For this review, take the finished solid that the model builds, in its own axes (mm). A direction names the side the tool comes from. Coordinates: 2 decimals unless noted, no trailing zeros. Loops run counter-clockwise (first coordinate to the right, second up) from the corner with the lowest first, then second, coordinate; pieces in that order, holes last. Notation, with made-up numbers: M 6.25,-8 L 13.25,-8 A32 cw 13.25,18 Z; hole C 79.5,63 d6. An arc over 180 degrees is marked long. Write each question's results on one line, items separated by ' | '. Start each with the question number.
```python
from build123d import *

# Parameters (mm, degrees)
EXTRUDE_1_DEPTH     = 39.9
SKETCH_2_R          = 1.5
CUT_EXTRUDE_1_DEPTH = 3
CHAMFER_1_SIZE      = 0.5


with BuildPart() as part:
    # 草图1 → 凸台-拉伸1 (new body)
    with BuildSketch(Plane(origin=(0, 0, 0), x_dir=(1, 0, 0), z_dir=(0, 1, 0))):
        Polygon((-10, 4), (-10, -4), (-4.5, -4), (-4.5, -2.84), (-3.55, -2.84), (-3.55, -1.36), (-4.5, -1.36), (-4.5, 0), (4.5, 0), (4.5, -1.36), (3.55, -1.36), (3.55, -2.84), (4.5, -2.84), (4.5, -4), (10, -4), (10, 4), align=None)
    extrude(amount=EXTRUDE_1_DEPTH)

    # 草图2 → 切除-拉伸1 (cut)
    with BuildSketch(Plane(origin=(0, 0, -4), x_dir=(-1, 0, 0), z_dir=(0, 0, -1))):
        with Locations((7.5, 27.95)):
            Circle(SKETCH_2_R)
        with Locations(Location((-7.5, 27.95, 0), (0, 0, 180))):
            Circle(SKETCH_2_R)
        with Locations(Location((7.5, 11.95, 0), (0, 0, 180))):
            Circle(SKETCH_2_R)
        with Locations((-7.5, 11.95)):
            Circle(SKETCH_2_R)
    extrude(amount=-CUT_EXTRUDE_1_DEPTH, mode=Mode.SUBTRACT)

    # 倒角1
    chamfer_1_edges = [part.edges().sort_by_distance(p)[0] for p in [
        (-10, 19.95, 4),
        (-10, 19.95, -4),
        (10, 19.95, -4),
        (10, 19.95, 4),
    ]]
    chamfer(chamfer_1_edges, length=CHAMFER_1_SIZE)


solid = part.part
```
Q1. To check wall thickness, follow line 1 along Y through (x, z) = (-7.5, -2.3); line 2 along X through (y, z) = (35, 1); line 3 along Z through (x, y) = (-3, 20). State the ranges of each line that lie inside material, in increasing order.
Q2. Take a section at C-C, the plane x = 7.5. Give the boundary of the cut face in (y, z), then the cut area to 3 significant figures.
Q3. For faces 4 (the face through (-3.55, 20, 2)), 5 (the face through (-8.69, 12.86, -2.52)), 6 (the face through (-4.5, 20, 1)), list the 3-axis set-ups (+Z, -Z, +X, -X, +Y, -Y) from which the entire face can be reached by the end or side of a thin tool; tool diameter is ignored.
Q4. Take a section at A-A, the plane z = -2.25. Give the boundary of the cut face in (x, y), then the cut area to 3 significant figures.
Q5. Insertion check: P1, Ø10, axis at x = -0.5, y = 21, coming from the +Z side; P2, Ø2.5, axis at x = -7.5, y = 11.95, coming from the -Z side. Each pin has a flat end and moves straight along its axis. Give the tip position at first contact, or say it passes through.
Q6. The part is to be moulded in two halves that separate along X. For faces 1 (the face through (7, 20, 4)), 2 (the face through (10, 20, 0)), 3 (the face through (-4.5, 20, 3)), say which applies: pulls with the +X half, pulls with the -X half, needs draft (parallel to the pull), parting line crosses it, or undercut.
Q7. Take a section at D-D, the plane y = 11. Give the boundary of the cut face in (x, z).
Q8. Take a section at B-B, the plane y = 24. Give the boundary of the cut face in (x, z).
Results:
1) line 1: 0 to 10.45, 13.45 to 26.45, 29.45 to 39.9 | line 2: -10 to -4.5, 4.5 to 10 | line 3: -4 to 0
2) outline: M 0,-4 L 10.45,-4 L 10.45,-1 L 13.45,-1 L 13.45,-4 L 26.45,-4 L 26.45,-1 L 29.45,-1 L 29.45,-4 L 39.9,-4 L 39.9,4 L 0,4 Z | area: 301 mm^2
3) face 4: +Z, +Y, -Y | face 5: -Z | face 6: +Y, -Y
4) outline: M -10,0 L 10,0 L 10,39.9 L -10,39.9 Z; hole C -7.5,11.95 d3; hole C -7.5,27.95 d3; hole C 7.5,11.95 d3; hole C 7.5,27.95 d3 | area: 770 mm^2
5) P1: z = 4 | P2: z = -1
6) face 1: needs draft | face 2: pulls with the +X half | face 3: undercut
7) outline: M -10,-3.5 L -9.5,-4 L -8.66,-4 L -8.66,-1 L -6.34,-1 L -6.34,-4 L 6.34,-4 L 6.34,-1 L 8.66,-1 L 8.66,-4 L 9.5,-4 L 10,-3.5 L 10,3.5 L 9.5,4 L 4.5,4 L 4.5,2.84 L 3.55,2.84 L 3.55,1.36 L 4.5,1.36 L 4.5,0 L -4.5,0 L -4.5,1.36 L -3.55,1.36 L -3.55,2.84 L -4.5,2.84 L -4.5,4 L -9.5,4 L -10,3.5 Z
8) outline: M -10,-3.5 L -9.5,-4 L 9.5,-4 L 10,-3.5 L 10,3.5 L 9.5,4 L 4.5,4 L 4.5,2.84 L 3.55,2.84 L 3.55,1.36 L 4.5,1.36 L 4.5,0 L -4.5,0 L -4.5,1.36 L -3.55,1.36 L -3.55,2.84 L -4.5,2.84 L -4.5,4 L -9.5,4 L -10,3.5 Z
